Print and shaded views of the part. All mm, measured from the part's lowest x, y and z. A direction names the side the tool comes from. Round coordinates to 2 decimals unless told otherwise and drop trailing zeros. Loops run counter-clockwise (first coordinate to the right, second up) from the corner with the lowest first, then second, coordinate; pieces in that order, holes last. Notation, with made-up numbers: (53, -28.75) -> (109, -28.75) arc R19 cw to (109, 7.25) -> close; hole circle Ø8 at (20.5, -25). An arc over 180 degrees is marked (long way). Use a Markdown table: item, result.
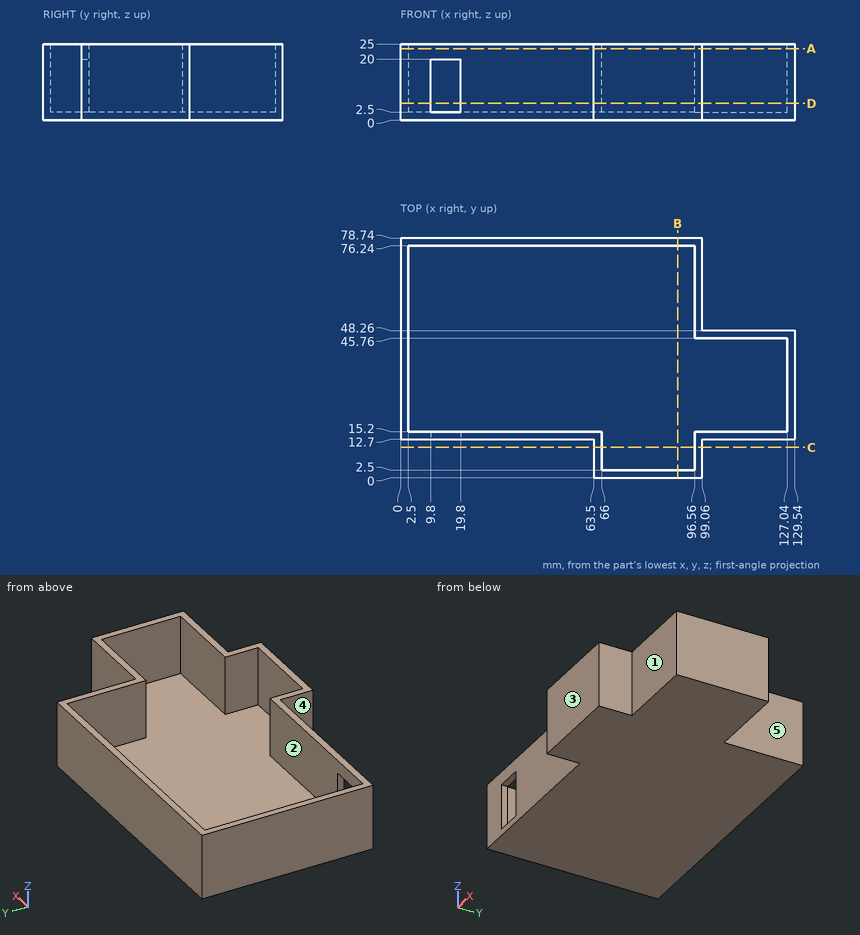
Q1. Band-saw the part on A-A, the plane z = 23.5. Give the cut face in (x, y).
Results list:
| item | result |
|---|---|
| outline | (0, 12.7) -> (63.5, 12.7) -> (63.5, 0) -> (99.06, 0) -> (99.06, 12.7) -> (129.54, 12.7) -> (129.54, 48.26) -> (99.06, 48.26) -> (99.06, 78.74) -> (0, 78.74) -> close; hole (2.5, 15.2) -> (66, 15.2) -> (66, 2.5) -> (96.56, 2.5) -> (96.56, 15.2) -> (127.04, 15.2) -> (127.04, 45.76) -> (96.56, 45.76) -> (96.56, 76.24) -> (2.5, 76.24) -> close |
Q2. Tool access for the marked faces 1, 2, 3, 4 and 5: list every direction of +Z, -Z, +X, -X, +Y, -Y with a clear straight run to the whole face (end or side of a thin tool).
Results list:
| item | result |
|---|---|
| face 1 | +Z, -Z, +X, -Y |
| face 2 | +Z |
| face 3 | +Z, -Z, +X, -X, -Y |
| face 4 | +Z, -Z, -X, -Y |
| face 5 | +Z, -Z, +X, +Y |
Q3. Band-saw the part on D-D, the plane z = 5.5. Give the cut face in (x, y).
Results list:
| item | result |
|---|---|
| outline | (0, 12.7) -> (9.8, 12.7) -> (9.8, 15.2) -> (2.5, 15.2) -> (2.5, 76.24) -> (96.56, 76.24) -> (96.56, 45.76) -> (127.04, 45.76) -> (127.04, 15.2) -> (96.56, 15.2) -> (96.56, 2.5) -> (66, 2.5) -> (66, 15.2) -> (19.8, 15.2) -> (19.8, 12.7) -> (63.5, 12.7) -> (63.5, 0) -> (99.06, 0) -> (99.06, 12.7) -> (129.54, 12.7) -> (129.54, 48.26) -> (99.06, 48.26) -> (99.06, 78.74) -> (0, 78.74) -> close |
Q4. Drill centre lines: L1, parallel to Y at x = 83.5, z = 5.5; L2, parallel to X at y = 4, z = 12.5; L3, parallel to X at y = 73.5, z = 16.75. Where is each one in solid material? Low to high. Write a range as from..to.
Results list:
| item | result |
|---|---|
| L1 | y = 0..2.5, 76.24..78.74 |
| L2 | x = 63.5..66, 96.56..99.06 |
| L3 | x = 0..2.5, 96.56..99.06 |
Q5. Band-saw the part on C-C, the plane y = 10. Give the cut face in (x, z).
Results list:
| item | result |
|---|---|
| outline | (63.5, 0) -> (99.06, 0) -> (99.06, 25) -> (96.56, 25) -> (96.56, 2.5) -> (66, 2.5) -> (66, 25) -> (63.5, 25) -> close |
Q6. Flat gauge pins, fed straight in: pin 1 (7 mm diameter, centred on x = 114.5, z = 18.5, fed in from +Y); pin 2 (4 mm diameter, centred on y = 9.5, z = 9, fed in from +X); pin 3 (1 mm diameter, centred on x = 44.5, y = 23, fed in from +Z); pin 4 (1 mm diameter, centred on x = 27, y = 11, fed in from -Z). Where does each tip first touch, or does it go through?
Results list:
| item | result |
|---|---|
| pin 1 | stops at y = 48.26 |
| pin 2 | stops at x = 99.06 |
| pin 3 | stops at z = 2.5 |
| pin 4 | passes through |
Q7. Band-saw the part on B-B, the plane x = 91. Give the cut face in (y, z), plus the area to 3 significant figures.
Results list:
| item | result |
|---|---|
| outline | (0, 0) -> (78.74, 0) -> (78.74, 25) -> (76.24, 25) -> (76.24, 2.5) -> (2.5, 2.5) -> (2.5, 25) -> (0, 25) -> close |
| area | 309 mm² |
